The listing builds one solid part. Answer for the finished solid, in the listing's coordinates (mm). Give positions to 0.01 mm unless a question says otherwise; leave off trailing zeros. Order: outer loops, then holes, each group sorted by start corner. A loop starts at its lowest first (then second) coordinate and runs counter-clockwise, first axis right, second up. Notation, with made-up numbers: M -23,16 L 28,16 A21 ccw 28,38 Z; hole C 36.25,57 d9. An arc over 180 degrees is marked long. Answer as a JSON object with one key per item and string values. Group by question number.
```python
from build123d import *

# Parameters (mm, degrees)
EXTRUDE_1_DEPTH          = 5
CUT_EXTRUDE_2_REACH      = 73.149
SKETCH_4_R               = 2
SKETCH_5_OUTSIDE_W       = 80.924
SKETCH_5_OUTSIDE_H       = 117.424
SKETCH_5_OUTSIDE_R       = 1.6
CUT_EXTRUDE_3_DEPTH      = 72.149490511
FILLET_1_R               = 6
FILLET_2_R               = 6
PATTERN_CIRCULAR_1_COUNT = 6


with BuildPart() as part:
    # 草圖1 → 填料-伸長1 (new body)
    with BuildSketch(Plane.XY):
        with BuildLine():
            Line((28.5, 65), (-28.5, 65))
            Line((-28.5, 65), (-28.5, 55))
            Line((-28.5, 55), (-28.5, 0))
            ThreePointArc((-28.5, 0), (-26.682182849, -10.015543839), (-21.46062327, -18.753443653))
            ThreePointArc((-21.46062327, -18.753443653), (0, -28.5), (21.46062327, -18.753443653))
            ThreePointArc((21.46062327, -18.753443653), (26.682182849, -10.015543839), (28.5, 0))
            Line((28.5, 0), (28.5, 55.020450743))
            Line((28.5, 55.020450743), (28.5, 65))
        make_face()
    extrude(amount=EXTRUDE_1_DEPTH)

    # 草圖4 → 除料-伸長2 (cut, up to next)
    with BuildSketch(Plane.XY.offset(5), mode=Mode.PRIVATE) as cut_extrude_2_sk1:
        with Locations((0, -15.5)):
            Circle(SKETCH_4_R)
    cut_extrude_2_tool1 = extrude(cut_extrude_2_sk1.sketch, amount=-CUT_EXTRUDE_2_REACH, mode=Mode.PRIVATE) & part.part
    cut_extrude_2 = cut_extrude_2_tool1.solids().sort_by_distance((0, -15.5, 5))[0]
    add(cut_extrude_2, mode=Mode.SUBTRACT)

    # 草圖5 outside → 除料-伸長3 (cut, through all)
    # profile 1 of 5: a face of its own
    with BuildSketch(Plane.XY.offset(5)):
        with Locations((0, 18.25)):
            Rectangle(SKETCH_5_OUTSIDE_W, SKETCH_5_OUTSIDE_H)
        with BuildLine():
            Line((28.5, 65), (-28.5, 65))
            Line((-28.5, 65), (-28.5, 0))
            ThreePointArc((-28.5, 0), (0, -28.5), (28.5, 0))
            Line((28.5, 0), (28.5, 65))
        make_face(mode=Mode.SUBTRACT)
    # profile 2 of 5: a face of its own
    with BuildSketch(Plane.XY.offset(5)):
        with Locations((22.5, 61)):
            Circle(SKETCH_5_OUTSIDE_R)
    # profile 3 of 5: a face of its own
    with BuildSketch(Plane.XY.offset(5)):
        with Locations((7.5, 61)):
            Circle(SKETCH_5_OUTSIDE_R)
    # profile 4 of 5: a face of its own
    with BuildSketch(Plane.XY.offset(5)):
        with Locations((-7.5, 61)):
            Circle(SKETCH_5_OUTSIDE_R)
    # profile 5 of 5: a face of its own
    with BuildSketch(Plane.XY.offset(5)):
        with Locations((-22.5, 61)):
            Circle(SKETCH_5_OUTSIDE_R)
    extrude(amount=-CUT_EXTRUDE_3_DEPTH, mode=Mode.SUBTRACT)

    # 圓角1
    fillet_1_edges = [part.edges().sort_by_distance(p)[0] for p in [
        (-28.5, 65, 2.5),
    ]]
    fillet(fillet_1_edges, radius=FILLET_1_R)

    # 圓角2
    fillet_2_edges = [part.edges().sort_by_distance(p)[0] for p in [
        (28.5, 65, 2.5),
    ]]
    fillet(fillet_2_edges, radius=FILLET_2_R)

    # 環狀複製排列1: 除料-伸長2 ×6 about axis
    pattern_circular_1_axis = Axis((0, 0, 0), (0, 0, 1))
    for i in range(1, PATTERN_CIRCULAR_1_COUNT):
        add(cut_extrude_2.rotate(pattern_circular_1_axis, i * 360 / PATTERN_CIRCULAR_1_COUNT), mode=Mode.SUBTRACT)


solid = part.part
```
Item 1: Section A-A (y = 7.75) is taken. Determine the outline of the cut face in (x, z).
Item 2: Section B-B (z = 1.8) is taken. Count the separate pieces of the cut face and the enclosed holes in it, and give its area (3 significant figures).
Item 3: Determine the mould class of faces 1 (the cylindrical face through (26.696, 63.289, 2.535)), 2 (the flat face through (-28.5, 30, 2)), 3 (the cylindrical face through (-14.9, 9.1, 2.5)) for opening direction Y: released by +Y, released by -Y, zero draft, split by the parting line, or undercut.
Item 4: Section D-D (x = -7.5) is taken. Determine the outline of the cut face in (y, z), and give its area (3 significant figures).
Item 5: Consider probe 1 along Y at (x, z) = (0, 3.35); probe 2 along Y at (x, z) = (-14, 1.3); probe 3 along X at (y, z) = (15.5, 2.25). Determine where each line is inside the solid, lowest interval first. Write a range as from..to.
Item 6: Section C-C (y = 61) is taken. Determine the outline of the cut face in (x, z).
Values found:
{
 "1": {"outline": "M -28.5,0 L -15.42,0 L -15.42,5 L -28.5,5 Z; M -11.42,0 L 11.42,0 L 11.42,5 L -11.42,5 Z; M 15.42,0 L 28.5,0 L 28.5,5 L 15.42,5 Z"},
 "2": {"separate pieces": "1", "enclosed holes": "10", "area": "4,860 mm^2"},
 "3": {"face 1": "released by +Y", "face 2": "zero draft", "face 3": "undercut"},
 "4": {"outline": "M -27.5,0 L 59.4,0 L 59.4,5 L -27.5,5 Z; M 62.6,0 L 65,0 L 65,5 L 62.6,5 Z", "area": "446 mm^2"},
 "5": {"probe 1": "y = -28.5..-17.5, -13.5..13.5, 17.5..65", "probe 2": "y = -24.82..-9.67, -5.83..5.83, 9.67..65", "probe 3": "x = -28.5..-2, 2..28.5"},
 "6": {"outline": "M -28.16,0 L -24.1,0 L -24.1,5 L -28.16,5 Z; M -20.9,0 L -9.1,0 L -9.1,5 L -20.9,5 Z; M -5.9,0 L 5.9,0 L 5.9,5 L -5.9,5 Z; M 9.1,0 L 20.9,0 L 20.9,5 L 9.1,5 Z; M 24.1,0 L 28.16,0 L 28.16,5 L 24.1,5 Z"}
}
